from build123d import *

# Parameters (mm, degrees)
BOSS_EXTRUDE1_DEPTH = 7
SKETCH2_R           = 1.6
CUT_EXTRUDE1_DEPTH  = 35.813215881
SKETCH3_R           = 3.1
CUT_EXTRUDE2_DEPTH  = 35.813215926
SKETCH4_R           = 3.1
CUT_EXTRUDE3_DEPTH  = 35.813215926
FILLET1_R           = 1.5


with BuildPart() as part:
    # Sketch1 → Boss-Extrude1 (new body)
    with BuildSketch(Plane(origin=(0, 0, 0), x_dir=(1, 0, 0), z_dir=(0, 1, 0))):
        with BuildLine():
            Line((3.5, -7.709447398), (3.5, -3.709447398))
            ThreePointArc((3.5, -3.709447398), (4.75081501, -1.85465812), (5.087489656, 0.357))
            Line((5.087489656, 0.357), (2.992640974, 30.21))
            ThreePointArc((2.992640974, 30.21), (0, 33), (-2.992640974, 30.21))
            Line((-2.992640974, 30.21), (-5.087489656, 0.357))
            ThreePointArc((-5.087489656, 0.357), (-4.75081501, -1.85465812), (-3.5, -3.709447398))
            Line((-3.5, -3.709447398), (-3.5, -7.709447398))
            Line((-3.5, -7.709447398), (-0.5, -7.709447398))
            Line((-0.5, -7.709447398), (-0.5, -3.059411708))
            ThreePointArc((-0.5, -3.059411708), (0, 3.1), (0.5, -3.059411708))
            Line((0.5, -3.059411708), (0.5, -7.709447398))
            Line((0.5, -7.709447398), (3.5, -7.709447398))
        make_face()
    extrude(amount=BOSS_EXTRUDE1_DEPTH)

    # Sketch2 → Cut-Extrude1 (cut, through all)
    with BuildSketch(Plane(origin=(3.5, 0, 0), x_dir=(0, 0, -1), z_dir=(1, 0, 0))):
        with Locations((-4.709447398, 3.5)):
            Circle(SKETCH2_R)
    extrude(amount=-CUT_EXTRUDE1_DEPTH, mode=Mode.SUBTRACT)

    # Sketch3 → Cut-Extrude2 (cut, through all)
    with BuildSketch(Plane(origin=(3.5, 0, 0), x_dir=(0, 0, -1), z_dir=(1, 0, 0))):
        with Locations((-4.709447398, 3.5)):
            Circle(SKETCH3_R)
    extrude(amount=CUT_EXTRUDE2_DEPTH, mode=Mode.SUBTRACT)

    # Sketch4 → Cut-Extrude3 (cut, through all)
    with BuildSketch(Plane.ZY.offset(3.5)):
        with Locations((4.709447398, 3.5)):
            Circle(SKETCH4_R)
    extrude(amount=CUT_EXTRUDE3_DEPTH, mode=Mode.SUBTRACT)

    # Fillet1
    # the kernel refuses this fillet: 1.5 mm, written as the material it takes off along each edge
    with BuildSketch(Plane(origin=(0, 0, 0), x_dir=(-0.9975469913743412, 0, -0.06999999999999885), z_dir=(0.06999999999999885, 0, -0.9975469913743412))) as fillet1_piece_1_section:
        with BuildLine():
            CenterArc((5.1 - FILLET1_R, FILLET1_R), FILLET1_R, 270, 90)
            Line((5.1 - FILLET1_R, 0), (5.1, 0))
            Line((5.1, 0), (5.1, FILLET1_R))
        make_face()
    fillet1_piece_1 = revolve(axis=Axis((0, 0, 0), (0, 1, 0)), revolution_arc=92.812679078, mode=Mode.PRIVATE)
    fillet1_piece_1 = split(fillet1_piece_1, bisect_by=Plane(origin=(-3.5, 0.37107605, 1.567580694), z_dir=(-1, 0, 0)), keep=Keep.TOP, mode=Mode.PRIVATE)
    add(fillet1_piece_1, mode=Mode.SUBTRACT)
    with BuildSketch(Plane(origin=(0, 0, 0), x_dir=(0.020965246222385766, 0, 0.9997802050705118), z_dir=(-0.9997802050705118, 0, 0.020965246222385766))) as fillet1_piece_2_section:
        with BuildLine():
            CenterArc((5.1 - FILLET1_R, FILLET1_R), FILLET1_R, 270, 90)
            Line((5.1, FILLET1_R), (5.1, 0))
            Line((5.1, 0), (5.1 - FILLET1_R, 0))
        make_face()
    fillet1_piece_2 = revolve(axis=Axis((0, 0, 0), (0, 1, 0)), revolution_arc=92.812679078, mode=Mode.PRIVATE)
    fillet1_piece_2 = split(fillet1_piece_2, bisect_by=Plane(origin=(3.5, 0.371076241, 1.567580599), z_dir=(1, 0, 0)), keep=Keep.TOP, mode=Mode.PRIVATE)
    add(fillet1_piece_2, mode=Mode.SUBTRACT)
    with BuildSketch(Plane(origin=(5.087489656, 0, -0.357), x_dir=(0, 1, 0), z_dir=(-0.06999999999999998, 0, -0.9975469913743412)), Plane(origin=(-2.992640974, 0, -30.21), x_dir=(0, 1, 0), z_dir=(-0.06999999999999998, 0, 0.9975469913743412)), Plane(origin=(-2.992640974, 7, -30.21), x_dir=(0.9975469913743412, 0, 0.06999999999999998), z_dir=(-0.06999999999999998, 0, 0.9975469913743412))) as fillet1_piece_3:
        with BuildLine():
            CenterArc((FILLET1_R, -FILLET1_R), FILLET1_R, 90, 90)
            Line((0, -FILLET1_R), (0, 0))
            Line((0, 0), (FILLET1_R, 0))
        make_face()
    extrude(amount=29.926409741, mode=Mode.SUBTRACT)
    with BuildSketch(Plane(origin=(0, 0, -30), x_dir=(0.9975469913743412, 0, -0.07000000000000023), z_dir=(0.07000000000000023, 0, 0.9975469913743412))) as fillet1_piece_4:
        with BuildLine():
            CenterArc((3 - FILLET1_R, FILLET1_R), FILLET1_R, 270, 90)
            Line((3, FILLET1_R), (3, 0))
            Line((3, 0), (3 - FILLET1_R, 0))
        make_face()
    revolve(axis=Axis((0, 0, -30), (0, 1, 0)), revolution_arc=171.972025564, mode=Mode.SUBTRACT)
    with BuildSketch(Plane(origin=(0, 7, 0), x_dir=(-0.9975469913743412, 0, -0.06999999999999885), z_dir=(0.06999999999999885, 0, -0.9975469913743412))) as fillet1_piece_5_section:
        with BuildLine():
            CenterArc((5.1 - FILLET1_R, -FILLET1_R), FILLET1_R, 0, 90)
            Line((5.1, -FILLET1_R), (5.1, 0))
            Line((5.1, 0), (5.1 - FILLET1_R, 0))
        make_face()
    fillet1_piece_5 = revolve(axis=Axis((0, 7, 0), (0, 1, 0)), revolution_arc=92.812679078, mode=Mode.PRIVATE)
    fillet1_piece_5 = split(fillet1_piece_5, bisect_by=Plane(origin=(-3.5, 6.628923944, 1.567580643), z_dir=(-1, 0, 0)), keep=Keep.TOP, mode=Mode.PRIVATE)
    add(fillet1_piece_5, mode=Mode.SUBTRACT)
    with BuildSketch(Plane(origin=(0, 7, 0), x_dir=(0.020965246222385686, 0, 0.9997802050705119), z_dir=(-0.9997802050705119, 0, 0.020965246222385686))) as fillet1_piece_6_section:
        with BuildLine():
            CenterArc((5.1 - FILLET1_R, -FILLET1_R), FILLET1_R, 0, 90)
            Line((5.1, -FILLET1_R), (5.1, 0))
            Line((5.1, 0), (5.1 - FILLET1_R, 0))
        make_face()
    fillet1_piece_6 = revolve(axis=Axis((0, 7, 0), (0, 1, 0)), revolution_arc=92.812679078, mode=Mode.PRIVATE)
    fillet1_piece_6 = split(fillet1_piece_6, bisect_by=Plane(origin=(3.5, 6.628923759, 1.567580599), z_dir=(1, 0, 0)), keep=Keep.TOP, mode=Mode.PRIVATE)
    add(fillet1_piece_6, mode=Mode.SUBTRACT)
    with BuildSketch(Plane(origin=(0, 7, -30), x_dir=(0.9975469913743412, 0, -0.07000000000000023), z_dir=(0.07000000000000023, 0, 0.9975469913743412))) as fillet1_piece_7:
        with BuildLine():
            CenterArc((3 - FILLET1_R, -FILLET1_R), FILLET1_R, 0, 90)
            Line((3, -FILLET1_R), (3, 0))
            Line((3, 0), (3 - FILLET1_R, 0))
        make_face()
    revolve(axis=Axis((0, 7, -30), (0, 1, 0)), revolution_arc=171.972025564, mode=Mode.SUBTRACT)
    with BuildSketch(Plane(origin=(5.087489656, 7, -0.357), x_dir=(0, -1, 0), z_dir=(-0.06999999999999998, 0, -0.9975469913743412))) as fillet1_piece_8:
        with BuildLine():
            CenterArc((FILLET1_R, FILLET1_R), FILLET1_R, 180, 90)
            Line((0, FILLET1_R), (0, 0))
            Line((0, 0), (FILLET1_R, 0))
        make_face()
    extrude(amount=29.926409741, mode=Mode.SUBTRACT)


solid = part.part
Source: CAD feature listing. Evaluate the final solid. Frame: model axes, mm. A direction names the side the tool comes from. Round coordinates to 2 decimals unless told otherwise and drop trailing zeros. Loops run counter-clockwise (first coordinate to the right, second up) from the corner with the lowest first, then second, coordinate; pieces in that order, holes last. Notation, with made-up numbers: (62.25, 5) - (94.25, 5) arc R37 cw to (94.25, 41) - close; hole circle Ø3 at (-18, -40). An arc over 180 degrees is marked (long way). Write item = value, one per line. Start each with the question number.
(1) Section query A-A, the plane y = 3.5. Output: boundary loops of the cut face in (x, z).
(2) Ray query, line 1 along X through (y, z) = (3.5, 0); line 2 along Z through (x, y) = (2.55, 3.5); line 3 along Z through (x, y) = (2.5, 3.5). Return the intervals inside material, ascending. Write a range as from..to.
(3) Pin query (flat end, axial travel): pin 1 (4 mm diameter, centred on y = 3.5, z = 4.71, fed in from +X); pin 2 (2.5 mm diameter, centred on y = 4.5, z = 5.5, fed in from -X); pin 3 (2 mm diameter, centred on y = 5.5, z = -15.5, fed in from -X); pin 4 (3.5 mm diameter, centred on x = 0, z = 0, fed in from -Y). Return the tip coordinate at first contact, or that it passes through.
(4) Pull-direction query (Z, two-part tool) for faces 5 (the face through (4.055, 3.472, -15.075)), 6 (the face through (-1.979, 3.981, 3.183)), 7 (the face through (-3.5, 3, 7)); classes: +Z half, -Z half, draft (parallel to the pull), parting line (faces both ways), or undercut.
(5) Set-up query: faces 1 (the face through (0, 3, -33)), 2 (the face through (-0.5, 3.5, 6.5)), 3 (the face through (3.5, 3, 7)), 4 (the face through (-4.01, 3.55, 1.61)). Return all of +Z, -Z, +X, -X, +Y, -Y with unobstructed straight access to the full face (end or side cutting, diameter ignored); none if empty.
Conclusion:
q1.outline = (-5.09, -0.36) - (-2.99, -30.21) arc R3 ccw to (2.99, -30.21) - (5.09, -0.36) arc R5.1 ccw to (4.84, 1.61) - (3.5, 1.61) - (3.5, 3.11) - (0.5, 3.11) - (0.5, 3.06) arc R3.1 cw (long way) to (-0.5, 3.06) - (-0.5, 3.11) - (-3.5, 3.11) - (-3.5, 1.61) - (-4.84, 1.61) arc R5.1 ccw to start; (-3.5, 6.31) - (-0.5, 6.31) - (-0.5, 7.71) - (-3.5, 7.71) - close; (0.5, 6.31) - (3.5, 6.31) - (3.5, 7.71) - (0.5, 7.71) - close
q2.line_1 = -5.1..-3.1, 3.1..5.1
q2.line_2 = -31.58..-1.76, 1.76..3.11, 6.31..7.71
q2.line_3 = -31.66..-1.83, 1.83..3.11, 6.31..7.71
q3.pin_1 = 3.5
q3.pin_2 = -3.5
q3.pin_3 = -4.1
q3.pin_4 = through
q4.face_5 = -Z half
q4.face_6 = undercut
q4.face_7 = draft
q5.face_1 = -Z, +Y, -Y
q5.face_2 = +Z, +Y, -Y
q5.face_3 = +Z, +X
q5.face_4 = +Z, -X
